Here's how the part is built. I have some questions about the finished solid (model axes, mm). Face numbers are marked on the shaded views. A direction names the side the tool comes from. Give positions to 0.01 mm unless a question says otherwise; leave off trailing zeros. Write each loop counter-clockwise with the first axis right and the second up, starting at its lowest first coordinate (ties: lowest second). Pieces come first, ordered by that corner, then holes. Notation, with made-up numbers: (49.25, -16) -> (76.25, -16) arc R25 cw to (76.25, 0) -> close; hole circle Ø2 at (19.25, 75.25). An arc over 180 degrees is marked (long way). Use CSV: the item, a comma, the result in double quotes. Start each with the question number.
(1) For pin 1 Ø5 at (y, z) = (-15, 21) entering from -X; pin 2 Ø3 at (y, z) = (5.5, 9) entering from +X; pin 3 Ø1 at (y, z) = (-16, 20) entering from +X, each with a flat end and sliding along its axis, tell me the tip position at first contact or that it passes through.
(2) Suppose I cut it at B-B on z = 13. List the corners of the cut face in (x, y) for me.
(3) If we mould it in two halves opening along X, with no side actions, what happens to the marked faces 3, 4, 5 and 6? For each: pulls with the +X half, pulls with the -X half, needs draft (parallel to the pull), parting line crosses it, or undercut.
(4) Suppose I cut it at A-A on z = 21. List the corners of the cut face in (x, y) for me.
(5) Suppose I cut it at C-C on x = 22. List the corners of the cut face in (y, z) for me, plus the area to 3 significant figures.
(6) I need wall thicknesses on L1, parallel to Y at x = 25, z = 15.5; L2, parallel to X at y = -6, z = 11.5; L3, parallel to Z at x = 12.5, y = -8. Which ranges of each line are inside material? Lowest first, please. Write a range as [from, to].
(7) Suppose I cut it at D-D on y = -10. List the corners of the cut face in (x, z) for me, plus the area to 3 significant figures.
(8) Which directions (+Z, -Z, +X, -X, +Y, -Y) give clear straight access to the entire face, cutting with the end or side of a thin tool? Please do the marked faces 1 and 2.
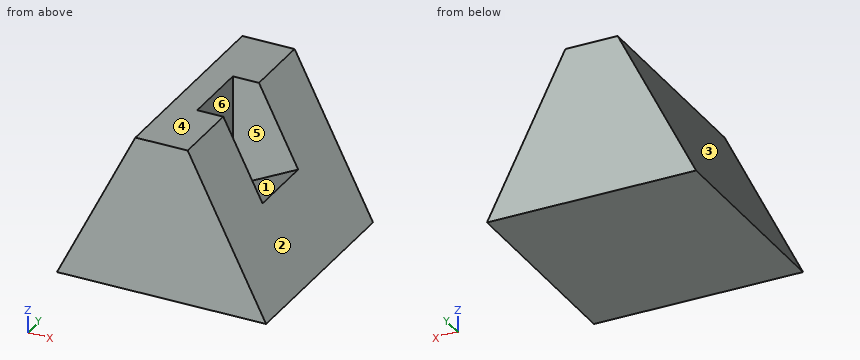
from build123d import *

# Parameters (mm, degrees)
F1_DEPTH = 20
F2_DEPTH = 6.6666666667


# Not quite as in the source:
# - a feature names something its author has since deleted; it is built from what else it names


with BuildPart() as f1:
    # F0 (on Front) → F1 (new body, symmetric)
    with BuildSketch(Plane.XZ):
        Polygon((15, 30), (0, 0), (40, 0), (32.5, 15), (20, 8.75), (20, 30), align=None)
        Polygon((20, 8.75), (32.5, 15), (25, 30), (20, 30), align=None)
    extrude(amount=F1_DEPTH, both=True)

    # F0 (on Front) → F2 (cut, symmetric)
    with BuildSketch(Plane.XZ):
        Polygon((20, 8.75), (32.5, 15), (25, 30), (20, 30), align=None)
    extrude(amount=F2_DEPTH, both=True, mode=Mode.SUBTRACT)


solid = f1.part
Geometry says:
1,pin 1,"x = 9.25"
1,pin 2,"x = 36.25"
1,pin 3,"x = 30.25"
2,outline,"(6.5, -20) -> (33.5, -20) -> (33.5, 20) -> (6.5, 20) -> close; hole (20, -6.67) -> (28.5, -6.67) -> (28.5, 6.67) -> (20, 6.67) -> close"
3,face 3,"pulls with the -X half"
3,face 4,"needs draft"
3,face 5,"undercut"
3,face 6,"undercut"
4,outline,"(10.5, -20) -> (29.5, -20) -> (29.5, -6.67) -> (20, -6.67) -> (20, 6.67) -> (29.5, 6.67) -> (29.5, 20) -> (10.5, 20) -> close"
5,outline,"(-20, 0) -> (20, 0) -> (20, 30) -> (6.67, 30) -> (6.67, 9.75) -> (-6.67, 9.75) -> (-6.67, 30) -> (-20, 30) -> close"
5,area,"930 mm²"
6,L1,"[-20, -6.67], [6.67, 20]"
6,L2,"[5.75, 20], [25.5, 34.25]"
6,L3,"[0, 25]"
7,outline,"(0, 0) -> (40, 0) -> (25, 30) -> (15, 30) -> close"
7,area,"750 mm²"
8,face 1,"+Z"
8,face 2,"+Z, +X, +Y, -Y"
